Geometry check sheet. Reference: drawing and pictorial views, mm from the part's lowest x, y, z. Round coordinates to 2 decimals unless told otherwise and drop trailing zeros. Order: outer loops, then holes, each group sorted by start corner. A loop starts at its lowest first (then second) coordinate and runs counter-clockwise, first axis right, second up.
(1) Sectioned sample at C-C, the plane y = 14. Enter the section's corners in (x, z), and give its area (3 significant figures).
(2) Depth check by flat-ended pin: pin 1 (3.5 mm diameter, centred on x = 5, y = 15, fed in from -Z). Enter the tip coordinate at first touch or a pass-through.
(3) Thickness scan on probe 1 along Y at (x, z) = (5, 5.75); probe 2 along Y at (x, z) = (5, 5.5); probe 3 along Z at (x, y) = (7.5, 5). Record the ranges inside material, lowest first.
(4) Mould release check, pull along Y, two halves, no side actions. Record for the marked faces 1, 2 and 3: released by +Y, released by -Y, zero draft, split by the parting line, or undercut.
(5) Sectioned sample at A-A, the plane x = 5. Enter the section's corners in (y, z), and give its area (3 significant figures).
(6) Sectioned sample at B-B, the plane z = 5. Enter the section's corners in (x, y).
(7) Sectioned sample at D-D, the plane z = 9. Enter the section's corners in (x, y).
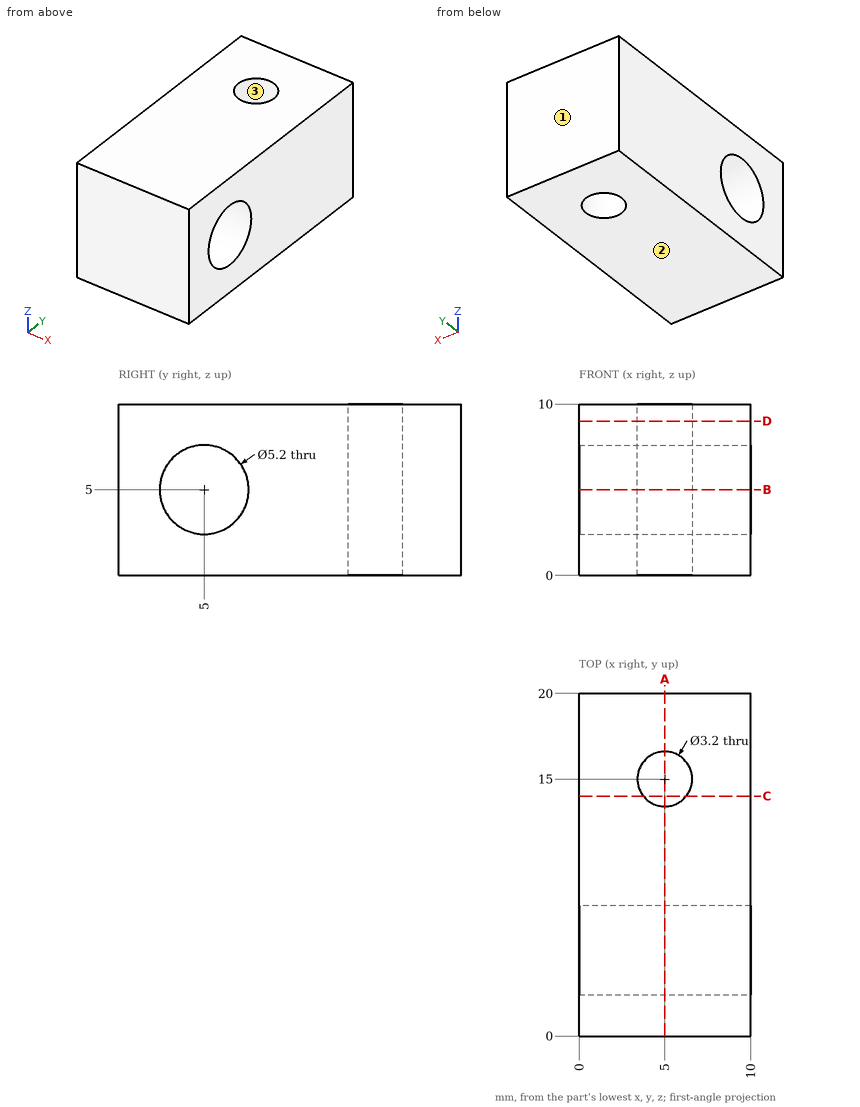
Derived:
1. outline: (0, 0) - (3.75, 0) - (3.75, 10) - (0, 10) - close; (6.25, 0) - (10, 0) - (10, 10) - (6.25, 10) - close
1. area: 75.0 mm2
2. pin 1: stops at z = 0
3. probe 1: y = 0 to 2.51, 7.49 to 13.4, 16.6 to 20
3. probe 2: y = 0 to 2.45, 7.55 to 13.4, 16.6 to 20
3. probe 3: z = 0 to 2.4, 7.6 to 10
4. face 1: released by +Y
4. face 2: zero draft
4. face 3: undercut
5. outline: (0, 0) - (13.4, 0) - (13.4, 10) - (0, 10) - close; (16.6, 0) - (20, 0) - (20, 10) - (16.6, 10) - close; hole circle Ø5.2 at (5, 5)
5. area: 147 mm2
6. outline: (0, 0) - (10, 0) - (10, 2.4) - (0, 2.4) - close; (0, 7.6) - (10, 7.6) - (10, 20) - (0, 20) - close; hole circle Ø3.2 at (5, 15)
7. outline: (0, 0) - (10, 0) - (10, 20) - (0, 20) - close; hole circle Ø3.2 at (5, 15)
